The listing builds one solid part. Answer for the finished solid, in the listing's coordinates (mm). Face numbers are marked on the shaded views. A direction names the side the tool comes from. Coordinates: 2 decimals unless noted, no trailing zeros. Loops run counter-clockwise (first coordinate to the right, second up) from the corner with the lowest first, then second, coordinate; pieces in that order, holes last. Notation, with made-up numbers: (-39, -36.5) - (0, -36.5) arc R16 cw to (0, -21.5) - close; hole circle Ø4 at (23.25, 19.25). An arc over 180 degrees is marked (long way). Return JSON: item names as keys, results as strings. Group by question number.
1. Each of these flat-tipped pins is pushed along its axis until it touches: P1, Ø1.5, axis at x = 2, y = 4, coming from the +Z side; P2, Ø1.5, axis at x = 1, y = 3.5, coming from the +Z side. Where does it stop, or does it pass through?
2. Section D-D (z = -4.5) is taken. Write down the section's boundary in (x, y), and give its area (3 significant figures).
3. The mould has two halves that part along Y. Classify the marked faces 1, 2 and 3: pulls with the +Y half, pulls with the -Y half, needs draft (parallel to the pull), parting line crosses it, or undercut.
4. Section A-A (y = 0) is taken. Write down the section's boundary in (x, z), and give its area (3 significant figures).
5. Section C-C (x = 1.1) is taken. Write down the section's boundary in (y, z), and give its area (3 significant figures).
6. Section B-B (z = 0) is taken. Write down the section's boundary in (x, y), and give its area (3 significant figures).
7. Find the intervals of material crossed by line 1 along Z through (x, y) = (1.3, 0); line 2 along Z through (x, y) = (0.85, 1.5); line 3 along Y through (x, z) = (1.6, 1.5), in increasing order.
8. Which of the six approach directions +Z, -Z, +X, -X, +Y, -Y give full straight-line access (tool end or side, diameter ignored) to the marked faces 4 and 5?
```python
from build123d import *

# Parameters (mm, degrees)
F0_R     = 2.9
F1_DEPTH = 3
F3_DEPTH = 3
F4_R     = 14.864409
F4_R_2   = 5.5
F5_DEPTH = 25.4


with BuildPart() as f1:
    # F0 (on Right) → F1 (new body)
    with BuildSketch(Plane.YZ):
        Polygon((0.84, 10.466346), (0, 12.5), (-0.838096, 10.465561), (-1.993439, 12.338134), (-2.494335, 10.1956), (-3.935098, 11.858594), (-4.085821, 9.663455), (-5.77469, 11.073799), (-5.571336, 8.88291), (-7.46457, 10.004076), (-6.912406, 7.874179), (-8.96097, 8.67713), (-8.074297, 6.663388), (-10.225136, 7.127329), (-9.026918, 5.281896), (-11.224325, 5.39481), (-9.745595, 3.765483), (-11.932659, 3.524446), (-10.211716, 2.153423), (-12.331793, 1.564677), (-10.413209, 0.487468), (-12.41139, -0.433738), (-10.344854, -1.189236), (-12.169387, -2.419043), (-10.008422, -2.833261), (-11.612053, -4.339818), (-9.412626, -4.402029), (-10.753822, -6.146318), (-8.572898, -5.85491), (-9.616923, -7.791753), (-7.510986, -7.154275), (-8.230799, -9.23351), (-6.254392, -8.26647), (-6.631351, -10.434246), (-4.835663, -9.162691), (-4.860004, -11.362863), (-3.291541, -9.819726), (-2.962635, -11.995311), (-1.66202, -10.220558), (-0.988385, -12.315209), (0.010698, -10.354806), (1.011615, -12.314273), (1.683289, -10.218992), (2.985565, -11.992527), (3.312434, -9.816635), (4.882341, -11.358303), (4.85594, -9.158155), (6.652818, -10.428028), (6.27383, -8.260606), (8.251141, -9.225795), (7.529382, -7.147235), (9.635915, -7.782742), (8.590078, -5.846877), (10.771274, -6.136242), (9.428445, -4.39321), (11.627813, -4.32894), (10.022772, -2.823885), (12.183349, -2.407644), (10.357664, -1.179545), (12.423493, -0.422113), (10.42445, 0.497221), (12.342025, 1.576227), (10.221398, 2.162987), (11.941057, 3.53562), (9.753768, 3.77461), (11.230972, 5.405321), (9.033671, 5.29035), (10.230161, 7.136903), (8.079758, 6.670949), (8.964545, 8.685521), (6.916733, 7.880652), (7.466903, 10.011065), (5.57472, 8.888127), (5.776023, 11.079206), (4.088475, 9.667282), (3.935697, 11.862278), (2.496491, 10.197936), (1.99359, 12.34), align=None)
        Circle(F0_R, mode=Mode.SUBTRACT)
    extrude(amount=F1_DEPTH)

    # F2 (on Right) → F3 (join)
    with BuildSketch(Plane.YZ):
        with BuildLine():
            ThreePointArc((2, -2.1), (2.9, 0), (2, 2.1))
            Line((2, 2.1), (2, -2.1))
        make_face()
    extrude(amount=F3_DEPTH)

    # F4 (on Right) → F5 (cut)
    with BuildSketch(Plane.YZ):
        Circle(F4_R)
        Circle(F4_R_2, mode=Mode.SUBTRACT)
    extrude(amount=F5_DEPTH, mode=Mode.SUBTRACT)


solid = f1.part
```
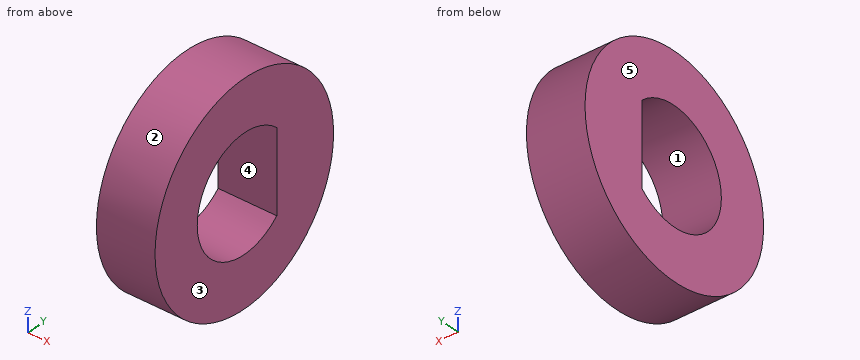
The answers:
{
 "1": {"P1": "stops at z = 4.44", "P2": "stops at z = 4.76"},
 "2": {"outline": "(0, -3.16) - (3, -3.16) - (3, 3.16) - (0, 3.16) - close", "area": "19.0 mm2"},
 "3": {"face 1": "undercut", "face 2": "parting line crosses it", "face 3": "needs draft"},
 "4": {"outline": "(0, -5.5) - (3, -5.5) - (3, -2.9) - (0, -2.9) - close; (0, 2.9) - (3, 2.9) - (3, 5.5) - (0, 5.5) - close", "area": "15.6 mm2"},
 "5": {"outline": "circle Ø11 at (0, 0); hole (2, -2.1) - (2, 2.1) arc R2.9 ccw (long way) to start", "area": "71.2 mm2"},
 "6": {"outline": "(0, -5.5) - (3, -5.5) - (3, -2.9) - (0, -2.9) - close; (0, 2) - (3, 2) - (3, 5.5) - (0, 5.5) - close", "area": "18.3 mm2"},
 "7": {"line 1": "z = -5.5 to -2.9, 2.9 to 5.5", "line 2": "z = -5.29 to -2.48, 2.48 to 5.29", "line 3": "y = -5.29 to -2.48, 2 to 5.29"},
 "8": {"face 4": "+X, -X", "face 5": "+Z, -Z, -X, +Y, -Y"}
}
